```python
from build123d import *

# Parameters (mm, degrees)
ESBO_O4_W                        = 2.25
ESBO_O4_H                        = 16
F_4_5_4_5_DIAMETER_HOLE2_D       = 4.5
F_4_5_4_5_DIAMETER_HOLE2_DEPTH   = 18
F_4_5_4_5_DIAMETER_HOLE2_TIP     = 1.351936393
ESBO_O12_R                       = 16
ESBO_O12_R_2                     = 9
RESSALTO_EXTRUS_O1_DEPTH         = 1
CHANFRO1_SIZE                    = 0.5
CHANFRO2_SIZE                    = 0.25
FURO_DE_DI_METRO_4_5_4_5_2_D     = 4.5
FURO_DE_DI_METRO_4_5_4_5_2_DEPTH = 8
FURO_DE_DI_METRO_4_5_4_5_2_TIP   = 1.351936393
ESBO_O18_R                       = 3.5
CORTE_EXTRUS_O4_DEPTH            = 0.5
ESBO_O20_R                       = 3.5
CORTE_EXTRUS_O5_DEPTH            = 0.5


# Read off the part's stored shape, not the designer's step: PadrãoCircular5
with BuildPart() as part:
    # Esboço1 → Revolução1 (revolve)
    with BuildSketch(Plane.XY, mode=Mode.PRIVATE) as revolu_o1_sk:
        Polygon((3, -9), (16, -9), (16, 5), (9, 5), (9, -5), (3, -5), align=None)
    revolve(revolu_o1_sk.sketch.rotate(Axis((0, -9, 0), (0, 1, 0)), 90), axis=Axis((0, -9, 0), (0, 1, 0)))

    # Esboço4 → Furo de diâmetro Ø4.5 (4.5)1 (revolve, cut)
    with BuildSketch(Plane(origin=(16, 0, 0), x_dir=(0, 0, -1), z_dir=(0, 1, 0))):
        with Locations((1.125, 8)):
            Rectangle(ESBO_O4_W, ESBO_O4_H)
    revolve(axis=Axis((22.35, 0, 0), (-1, 0, 0)), mode=Mode.SUBTRACT)

    # Ø4.5 (4.5) Diameter Hole2
    with Locations(Plane(origin=(-13.856406461, 0, -8), x_dir=(0, -1, 0), z_dir=(-0.8660254037844364, 0, -0.5000000000000041))):
        with Locations((0, 0)):
            Hole(F_4_5_4_5_DIAMETER_HOLE2_D / 2, depth=F_4_5_4_5_DIAMETER_HOLE2_DEPTH)
            with Locations((0, 0, -(F_4_5_4_5_DIAMETER_HOLE2_DEPTH + F_4_5_4_5_DIAMETER_HOLE2_TIP / 2))):  # 118° drill point
                Cone(0, F_4_5_4_5_DIAMETER_HOLE2_D / 2, F_4_5_4_5_DIAMETER_HOLE2_TIP, mode=Mode.SUBTRACT)

    # Esboço12 → Ressalto-extrusão1 (add)
    with BuildSketch(Plane(origin=(0, 5, 0), x_dir=(1, 0, 0), z_dir=(0, 1, 0))):
        with Locations(Location((0, 0, 0), (0, 0, 90))):
            Circle(ESBO_O12_R)
        with Locations(Location((0, 0, 0), (0, 0, 90))):
            Circle(ESBO_O12_R_2, mode=Mode.SUBTRACT)
    extrude(amount=RESSALTO_EXTRUS_O1_DEPTH)

    # Esboço13 → Furo roscado de M3x0.51 (revolve, cut)
    with BuildSketch(Plane(origin=(11.328847338, 6, -5.282728272), x_dir=(0, 0, 1), z_dir=(1, 0, 0))):
        Polygon((0, 0), (0, 10.751075774), (1.25, 10), (1.25, 0), align=None)
    revolve(axis=Axis((11.328847338, 12.35, -5.282728272), (0, -1, 0)), mode=Mode.SUBTRACT)

    # PadrãoCircular5 outline → PadrãoCircular5 (revolve, cut)
    with BuildSketch(Plane(origin=(5.282728272, 0, 11.328847338), x_dir=(1, 0, 0), z_dir=(0, 0, 1))):
        Polygon((0, 6), (0, -4.751075774), (1.25, -4), (1.25, 6), align=None)
    revolve(axis=Axis((5.282728272, 0, 11.328847338), (0, 1, 0)), mode=Mode.SUBTRACT)

    # Padr_oCircular5 2 outline → Padr_oCircular5 2 (revolve, cut)
    with BuildSketch(Plane(origin=(-11.328847338, 0, 5.282728272), x_dir=(1, 0, 0), z_dir=(0, 0, 1))):
        Polygon((0, 6), (0, -4.751075774), (1.25, -4), (1.25, 6), align=None)
    revolve(axis=Axis((-11.328847338, 0, 5.282728272), (0, 1, 0)), mode=Mode.SUBTRACT)

    # Padr_oCircular5 3 outline → Padr_oCircular5 3 (revolve, cut)
    with BuildSketch(Plane(origin=(-5.282728272, 0, -11.328847338), x_dir=(1, 0, 0), z_dir=(0, 0, 1))):
        Polygon((0, 6), (0, -4.751075774), (1.25, -4), (1.25, 6), align=None)
    revolve(axis=Axis((-5.282728272, 0, -11.328847338), (0, 1, 0)), mode=Mode.SUBTRACT)

    # Chanfro1
    chanfro1_edges = [part.edges().sort_by_distance(p)[0] for p in [
        (0, -5, 3),
    ]]
    chamfer(chanfro1_edges, length=CHANFRO1_SIZE)

    # Chanfro2
    chanfro2_edges = [part.edges().sort_by_distance(p)[0] for p in [
        (0, 6, 9),
    ]]
    chamfer(chanfro2_edges, length=CHANFRO2_SIZE)

    # Furo de diâmetro Ø4.5 (4.5)2
    with Locations(Plane(origin=(-16, 0, 0), x_dir=(0, 0, -1), z_dir=(-1, 0, 0))):
        with Locations((0, 0)):
            Hole(FURO_DE_DI_METRO_4_5_4_5_2_D / 2, depth=FURO_DE_DI_METRO_4_5_4_5_2_DEPTH)
            with Locations((0, 0, -(FURO_DE_DI_METRO_4_5_4_5_2_DEPTH + FURO_DE_DI_METRO_4_5_4_5_2_TIP / 2))):  # 118° drill point
                Cone(0, FURO_DE_DI_METRO_4_5_4_5_2_D / 2, FURO_DE_DI_METRO_4_5_4_5_2_TIP, mode=Mode.SUBTRACT)

    # Esboço18 → Corte-extrusão4 (cut)
    with BuildSketch(Plane(origin=(-16, 0, 0), x_dir=(0, -1, 0), z_dir=(-1, 0, 0))):
        with Locations(Location((0, 0, 0), (0, 0, 90))):
            Circle(ESBO_O18_R)
    corte_extrus_o4 = extrude(amount=-CORTE_EXTRUS_O4_DEPTH, mode=Mode.SUBTRACT)

    # Esboço20 → Corte-extrusão5 (cut)
    with BuildSketch(Plane(origin=(-13.856406461, 0, -8), x_dir=(0, -1, 0), z_dir=(-0.8660254037844364, 0, -0.5000000000000041))):
        with Locations(Location((0, 0, 0), (0, 0, 90))):
            Circle(ESBO_O20_R)
    extrude(amount=-CORTE_EXTRUS_O5_DEPTH, mode=Mode.SUBTRACT)

    # Espelhar1: Corte-extrusão4 across plane
    add(corte_extrus_o4.mirror(Plane(origin=(0, 0, 0), x_dir=(0, 0, 1), z_dir=(1, 0, 0))), mode=Mode.SUBTRACT)


solid = part.part
```
The model under review builds one solid part; all positions refer to its coordinate system, in mm. A direction names the side the tool comes from. Round coordinates to 2 decimals unless told otherwise and drop trailing zeros. Order: outer loops, then holes, each group sorted by start corner. A loop starts at its lowest first (then second) coordinate and runs counter-clockwise, first axis right, second up. Notation, with made-up numbers: (78.25, 16) -> (86.25, 16) arc R24 cw to (86.25, 35) -> close; hole circle Ø9 at (68, -14). An arc over 180 degrees is marked (long way). Use a Markdown table: item, result.
Q1. We need section C-C on y = 1. Write out the cut boundary in (x, z), then the cut area to 3 significant figures.
Values:
| item | result |
|---|---|
| outline | (-15.64, -3.35) arc R16 ccw to (-15.23, -4.92) -> (-15.1, -4.85) -> (-14.43, -6) -> (-8.6, -2.64) arc R9 cw to (-8.77, -2.02) -> (-15.5, -2.02) -> (-15.5, -3.35) -> close; (-15.64, 3.35) -> (-15.5, 3.35) -> (-15.5, 2.02) -> (-8.77, 2.02) arc R9 cw to (8.77, 2.02) -> (15.5, 2.02) -> (15.5, 3.35) -> (15.64, 3.35) arc R16 ccw to start; (-12.42, -9.5) -> (-11.75, -10.65) -> (-11.87, -10.73) arc R16 ccw to (15.64, -3.35) -> (15.5, -3.35) -> (15.5, -2.02) -> (8.77, -2.02) arc R9 cw to (-6.59, -6.13) -> close; hole circle Ø2.5 at (-11.33, 5.28); hole circle Ø2.5 at (-5.28, -11.33); hole circle Ø2.5 at (5.28, 11.33); hole circle Ø2.5 at (11.33, -5.28) |
| area | 443 mm^2 |
Q2. Clearance check with flat-ended pins moving along their axes: P1, Ø3, axis at y = 1, z = 12, coming from the +X side; P2, Ø5, axis at x = -8.5, y = -6.5, coming from the +Z side; P3, Ø3.5, axis at x = 0, z = 0, coming from the +Y side; P4, Ø1, axis at x = 3.5, y = -3.5, coming from the -Z side. State where each tip first meets the part, or that it passes through.
Values:
| item | result |
|---|---|
| P1 | stops at x = 12.07 |
| P2 | stops at z = 14.83 |
| P3 | passes through |
| P4 | stops at z = -15.72 |
Q3. We need section D-D on y = 4.75. Write out the cut boundary in (x, z), then the cut area to 3 significant figures.
Values:
| item | result |
|---|---|
| outline | circle Ø32 at (0, 0); hole circle Ø2.5 at (-11.33, 5.28); hole circle Ø18 at (0, 0); hole circle Ø2.5 at (-5.28, -11.33); hole circle Ø2.5 at (5.28, 11.33); hole circle Ø2.5 at (11.33, -5.28) |
| area | 530 mm^2 |
Q4. Mouldability with a two-part tool opening along X and no side actions: class faces 1 (the flat face through (-0.2, -9, 3.3)), 2 (the cylindrical face through (15.62, -1.39, 3.47)), 3 (the conical face through (11.264, -4.621, -5.076)) as +X half, -X half, draft (parallel to the pull), parting line (faces both ways), or undercut.
Values:
| item | result |
|---|---|
| face 1 | draft |
| face 2 | parting line |
| face 3 | undercut |
Q5. Tool access review of faces 4 (the cylindrical face through (-12.06, -2.23, -0.29)), 5 (the cylindrical face through (-5.554, 1.07, -10.109)): name each direction out of +Z, -Z, +X, -X, +Y, -Y from which nothing blocks a thin tool from reaching the whole face with its end or side.
Values:
| item | result |
|---|---|
| face 4 | +X, -X |
| face 5 | +Y |
Q6. We need section A-A on z = 0. State how many separate pieces and enclosed holes the cut face has, then the cut area to 3 significant figures.
Values:
| item | result |
|---|---|
| separate pieces | 4 |
| enclosed holes | 0 |
| area | 192 mm^2 |
Q7. For line 1 (Z direction, x = 5.5, y = -2); line 2 (Y direction, x = -13.5, z = -8); line 3 (Y direction, x = -12, z = 0), list the stretches that pass through material, from the lowest coordinate up.
Values:
| item | result |
|---|---|
| line 1 | z = -15.02 to -7.12, 7.12 to 10.1, 12.56 to 15.02 |
| line 2 | y = -9 to -3.5, 3.5 to 6 |
| line 3 | y = -9 to -2.25, 2.25 to 6 |
Q8. We need section B-B on x = 0. Write out the cut boundary in (y, z).
Values:
| item | result |
|---|---|
| outline | (-9, -16) -> (6, -16) -> (6, -9.25) -> (5.75, -9) -> (-5, -9) -> (-5, -3.5) -> (-5.5, -3) -> (-9, -3) -> close; (-9, 3) -> (-5.5, 3) -> (-5, 3.5) -> (-5, 9) -> (5.75, 9) -> (6, 9.25) -> (6, 16) -> (-9, 16) -> close |
